Geometry: final body of the model. Coordinates: model frame, mm. A direction names the side the tool comes from. Coordinates: 2 decimals unless noted, no trailing zeros. Write each loop counter-clockwise with the first axis right and the second up, starting at its lowest first coordinate (ties: lowest second). Pieces come first, ordered by that corner, then holes. Notation, with made-up numbers: (-30.5, 47.5) - (-12.5, 47.5) arc R34 ccw to (-12.5, 83.5) - close; hole circle Ø11 at (4.25, 11.5). An arc over 180 degrees is marked (long way). Answer as a JSON object with one key per item and string values. Group by question number.
Item 1: First-contact query: pin 1 Ø8 at (x, y) = (8.5, -23) entering from +Z. Flat tip, straight axial feed; report the tip coordinate or a pass-through.
Item 2: Line query: line 1 along Z through (x, y) = (3.75, -2.5). Output: solid intervals per line, ascending. Write a range as from..to.
Item 3: Mould query, pull axis X, two halves, no side actions, for faces 3 (the flat face through (0, 6, 24)), 4 (the flat face through (-5.08, 6, -10)), 5 (the flat face through (-3, 6, 27.354)). Classes: pulls with the +X half, pulls with the -X half, needs draft (parallel to the pull), parting line crosses it, or undercut.
Item 4: Section B-B on x = 10. Return loops of the section in (y, z), and give its area (3 significant figures).
Item 5: Section A-A on y = -13. Return loops of the section in (x, z).
Item 6: Set-up query: faces 1 (the flat face through (15.494, 6, 24)), 2 (the flat face through (20.32, 6, -10)). Return all of +Z, -Z, +X, -X, +Y, -Y with unobstructed straight access to the full face (end or side cutting, diameter ignored); none if empty.
```python
from build123d import *

# Parameters (mm, degrees)
F0_W     = 101.6
F0_H     = 6.21665
F0_H_2   = 69.98335
F1_DEPTH = 5.08
F2_DEPTH = 15.494
F3_START = 15.494
F3_DEPTH = 4.826


with BuildPart() as f1:
    # F0 (on Right) → F1 (new body)
    with BuildSketch(Plane.YZ):
        with Locations((6.5453828692, 24.245519595)):
            Rectangle(F0_W, F0_H)
        with Locations((6.5453828692, -13.854480405)):
            Rectangle(F0_W, F0_H_2)
    extrude(amount=-F1_DEPTH)

    # F0 (on Right) → F2 (join)
    with BuildSketch(Plane.YZ):
        with Locations((6.5453828692, -13.854480405)):
            Rectangle(F0_W, F0_H_2)
    extrude(amount=F2_DEPTH)

    # F0 (on Right) → F3 (join)
    with BuildSketch(Plane.YZ.offset(F3_START)):
        with Locations((6.5453828692, 24.245519595)):
            Rectangle(F0_W, F0_H)
        with Locations((6.5453828692, -13.854480405)):
            Rectangle(F0_W, F0_H_2)
    extrude(amount=F3_DEPTH)


solid = f1.part
```
Checks:
{
 "1": {"pin 1": "z = 21.14"},
 "2": {"line 1": "-48.85..21.14"},
 "3": {"face 3": "undercut", "face 4": "pulls with the -X half", "face 5": "needs draft"},
 "4": {"outline": "(-44.25, -48.85) - (57.35, -48.85) - (57.35, 21.14) - (-44.25, 21.14) - close", "area": "7,110 mm^2"},
 "5": {"outline": "(-5.08, -48.85) - (20.32, -48.85) - (20.32, 27.35) - (15.49, 27.35) - (15.49, 21.14) - (0, 21.14) - (0, 27.35) - (-5.08, 27.35) - close"},
 "6": {"face 1": "+Z, +Y, -Y", "face 2": "+Z, -Z, +X, +Y, -Y"}
}
